```python
from build123d import *

# Parameters (mm, degrees)
F0_R     = 4
F1_DEPTH = 11
F2_DEPTH = 3
F3_DEPTH = 5
F4_R     = 3


# Not quite as in the source:
# - a feature names something its author has since deleted; it is built from what else it names


with BuildPart() as f1:
    # F0 (on Top) → F1 (new body)
    with BuildSketch(Plane.XY):
        with Locations((-10.5441558773, 10.5441558773)):
            Circle(F0_R)
    extrude(amount=F1_DEPTH)

    # F0 (on Top) → F2 (join)
    with BuildSketch(Plane.XY):
        with BuildLine():
            ThreePointArc((-30.0251262658, 1.75), (-30.5376893988, 0.5125631329), (-31.7751262658, 0))
            Line((-31.7751262658, 0), (-1.7499999988, 0))
            ThreePointArc((-1.7499999988, 0), (-2.9874368675, 2.9874368666), (0, 1.75))
            Line((0, 1.75), (0, 31.7751262658))
            ThreePointArc((0, 31.7751262658), (-2.4196959983, 30.1583370805), (-2.9874368799, 33.0125631201))
            Line((-2.9874368799, 33.0125631201), (-33.0125631516, 2.9874368484))
            ThreePointArc((-33.0125631516, 2.9874368484), (-31.1054302714, 3.3667891869), (-30.0251262658, 1.75))
        make_face()
        Polygon((-3, 3), (-28.7573593129, 3), (-3, 28.7573593129), align=None, mode=Mode.SUBTRACT)
        Polygon((-3, 28.7573593129), (-28.7573593129, 3), (-3, 3), align=None)
        with Locations((-10.5441558773, 10.5441558773)):
            Circle(F0_R, mode=Mode.SUBTRACT)
        with BuildLine():
            ThreePointArc((-33.0125631516, 2.9874368484), (-33.3919154427, 1.0803039812), (-31.7751262658, 0))
            ThreePointArc((-31.7751262658, 0), (-30.5376893988, 0.5125631329), (-30.0251262658, 1.75))
            ThreePointArc((-30.0251262658, 1.75), (-31.1054302714, 3.3667891869), (-33.0125631516, 2.9874368484))
        make_face()
        with BuildLine():
            ThreePointArc((0, 1.75), (-2.9874368675, 2.9874368666), (-1.7499999988, 0))
            ThreePointArc((-1.7499999988, 0), (-0.5125631325, 0.5125631334), (0, 1.75))
        make_face()
        with BuildLine():
            ThreePointArc((0, 31.7751262658), (-1.0803040017, 33.3919154512), (-2.9874368799, 33.0125631201))
            ThreePointArc((-2.9874368799, 33.0125631201), (-2.4196959983, 30.1583370805), (0, 31.7751262658))
        make_face()
    extrude(amount=F2_DEPTH)

    # F0 (on Top) → F3 (join)
    with BuildSketch(Plane.XY):
        with BuildLine():
            ThreePointArc((-30.0251262658, 1.75), (-30.5376893988, 0.5125631329), (-31.7751262658, 0))
            Line((-31.7751262658, 0), (-1.7499999988, 0))
            ThreePointArc((-1.7499999988, 0), (-2.9874368675, 2.9874368666), (0, 1.75))
            Line((0, 1.75), (0, 31.7751262658))
            ThreePointArc((0, 31.7751262658), (-2.4196959983, 30.1583370805), (-2.9874368799, 33.0125631201))
            Line((-2.9874368799, 33.0125631201), (-33.0125631516, 2.9874368484))
            ThreePointArc((-33.0125631516, 2.9874368484), (-31.1054302714, 3.3667891869), (-30.0251262658, 1.75))
        make_face()
        Polygon((-3, 3), (-28.7573593129, 3), (-3, 28.7573593129), align=None, mode=Mode.SUBTRACT)
        with BuildLine():
            ThreePointArc((0, 1.75), (-2.9874368675, 2.9874368666), (-1.7499999988, 0))
            ThreePointArc((-1.7499999988, 0), (-0.5125631325, 0.5125631334), (0, 1.75))
        make_face()
        with BuildLine():
            ThreePointArc((0, 31.7751262658), (-1.0803040017, 33.3919154512), (-2.9874368799, 33.0125631201))
            ThreePointArc((-2.9874368799, 33.0125631201), (-2.4196959983, 30.1583370805), (0, 31.7751262658))
        make_face()
        with BuildLine():
            ThreePointArc((-33.0125631516, 2.9874368484), (-33.3919154427, 1.0803039812), (-31.7751262658, 0))
            ThreePointArc((-31.7751262658, 0), (-30.5376893988, 0.5125631329), (-30.0251262658, 1.75))
            ThreePointArc((-30.0251262658, 1.75), (-31.1054302714, 3.3667891869), (-33.0125631516, 2.9874368484))
        make_face()
    extrude(amount=-F3_DEPTH)

    # F4
    f4_edges = [f1.edges().sort_by_distance(p)[0] for p in [
        (-14.544156, 10.544156, 11),
    ]]
    fillet(f4_edges, radius=F4_R)


solid = f1.part
```
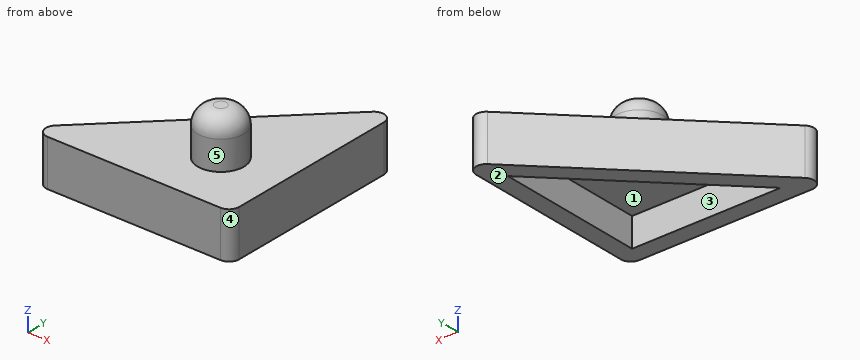
Geometry check sheet. Reference: the model listing, model coordinates, mm. Face numbers are marked on the shaded views. A direction names the side the tool comes from. Round coordinates to 2 decimals unless told otherwise and drop trailing zeros. Loops run counter-clockwise (first coordinate to the right, second up) from the corner with the lowest first, then second, coordinate; pieces in that order, holes last. Notation, with made-up numbers: (74, 76) - (104, 76) arc R23 ccw to (104, 111) - close; hole circle Ø4 at (25, -3.75). An arc over 180 degrees is marked (long way). Write each question's results on one line, items separated by ' | '. Start each with the question number.
Q1. Cross-section at B-B on x = -19. Enter the section's corners in (y, z), and give its area (3 significant figures).
Q2. Access from +Z, -Z, +X, -X, +Y, -Y to the whole of each face (thin tool, end or side, straight path). Record for the marked faces 1 and 2.
Q3. Thickness scan on line 1 (Z direction, x = -7.5, y = 18.5); line 2 (X direction, y = 22, z = -4.5); line 3 (Y direction, x = -12, z = -1.25). Record the ranges inside material, lowest first. Write a range as [from, to].
Q4. Cross-section at A-A on z = 1. Enter the section's corners in (x, y).
Q5. Release check for a two-part mould opening along Y. For the marked faces 3, 4 and 5 record: +Y half, -Y half, draft (parallel to the pull), parting line (faces both ways), or undercut.
Q6. Gauge pin test, flat ends, axial feed: P1, Ø10, axis at x = -25, y = 12.5, coming from the +Z side; P2, Ø4, axis at y = 15.5, z = -2, coming from the -X side; P3, Ø5.5, axis at y = 20.5, z = -1.5, coming from the -X side. Record the tip position at first contact, or that the pin passes through.
Q7. Cross-section at C-C on y = 16. Enter the section's corners in (x, z).
Q8. Cross-section at D-D on x = -30. Enter the section's corners in (y, z).
Answers below:
1) outline: (0, -5) - (3, -5) - (3, 0) - (12.76, 0) - (12.76, -5) - (17, -5) - (17, 3) - (0, 3) - close | area: 87.2 mm²
2) face 1: -Z | face 2: -Z, +X, -X, +Y, -Y
3) line 1: z = [0, 3] | line 2: x = [-14, -9.76], [-3, 0] | line 3: y = [0, 3], [19.76, 24]
4) outline: (-33.01, 2.99) arc R1.75 ccw to (-31.78, 0) - (-1.75, 0) arc R1.75 ccw to (0, 1.75) - (0, 31.78) arc R1.75 ccw to (-2.99, 33.01) - close
5) face 3: undercut | face 4: -Y half | face 5: parting line
6) P1: stops at z = 3 | P2: stops at x = -22.5 | P3: stops at x = -18.25
7) outline: (-20, -5) - (-15.76, -5) - (-15.76, 0) - (-3, 0) - (-3, -5) - (0, -5) - (0, 3) - (-20, 3) - close
8) outline: (0, -5) - (6, -5) - (6, 3) - (0, 3) - close
